Autodesk Inventor part; units mm, degrees
ref_plane "YZ Plane" through (0, 0, 0) normal (1, 0, 0) x (0, 1, 0)
ref_plane "XZ Plane" through (0, 0, 0) normal (0, 1, 0) x (-1, 0, 0)
ref_plane "XY Plane" through (0, 0, 0) normal (0, 0, 1) x (1, 0, 0)
sketch "Boceto1" plane through (0, 0, 0) normal (0, 1, 0) x (-1, 0, 0)
  line L0 (0, 0) -> (88.9, 0)
  line L1 (88.9, 0) -> (88.9, -139.7)
  line L2 (88.9, -139.7) -> (0, -139.7)
  line L3 (0, -139.7) -> (0, 0)
  circle A0 centre (60.325, -25.4) radius 3.9688
  circle A1 centre (60.325, -114.3) radius 3.9688
  circle A2 centre (28.575, -25.4) radius 3.9687
  circle A3 centre (28.575, -114.3) radius 3.9687
  line L4 (88.9, 0) -> (94.4562, 0)
  line L5 (94.4562, 0) -> (94.4562, -12.7)
  line L6 (94.4562, -12.7) -> (88.9, -12.7)
  line L7 (88.9, -12.7) -> (88.9, 0)
  line L8 (88.9, -139.7) -> (94.4563, -139.7)
  line L9 (94.4563, -139.7) -> (94.4563, -127)
  line L10 (94.4563, -127) -> (88.9, -127)
  line L11 (88.9, -127) -> (88.9, -139.7)
  line L12 (0, 0) -> (-5.5563, 0)
  line L13 (-5.5563, 0) -> (-5.5563, -12.7)
  line L14 (-5.5563, -12.7) -> (0, -12.7)
  line L15 (0, -12.7) -> (0, 0)
  line L16 (0, -139.7) -> (-5.5562, -139.7)
  line L17 (-5.5562, -139.7) -> (-5.5562, -127)
  line L18 (-5.5562, -127) -> (0, -127)
  line L19 (0, -127) -> (0, -139.7)
  line L20 (88.9, -63.5) -> (94.4562, -63.5)
  line L21 (94.4562, -63.5) -> (94.4562, -76.2)
  line L22 (94.4562, -76.2) -> (88.9, -76.2)
  line L23 (88.9, -76.2) -> (88.9, -63.5)
  line L24 (0, -63.5) -> (-5.5563, -63.5)
  line L25 (-5.5563, -63.5) -> (-5.5563, -76.2)
  line L26 (-5.5563, -76.2) -> (0, -76.2)
  line L27 (0, -76.2) -> (0, -63.5)
  dimension "d0" = 88.9
  dimension "d1" = 139.7
  dimension "d2" = 7.9375
  dimension "d3" = 7.9375
  dimension "d4" = 7.9375
  dimension "d5" = 7.9375
  dimension "d6" = 88.9
  dimension "d7" = 28.575
  dimension "d8" = 28.575
  dimension "d9" = 28.575
  dimension "d10" = 28.575
  dimension "d11" = 25.4
  dimension "d12" = 25.4
  dimension "d13" = 88.9
  dimension "d17" = 5.5563
  dimension "d18" = 12.7
  dimension "d19" = 5.5563
  dimension "d20" = 12.7
  dimension "d21" = 5.5563
  dimension "d22" = 12.7
  dimension "d23" = 5.5563
  dimension "d24" = 12.7
  dimension "d25" = 5.5563
  dimension "d26" = 12.7
  dimension "d27" = 5.5563
  dimension "d28" = 12.7
  dimension "d29" = 63.5
  dimension "d30" = 63.5
extrude "Extrusión1" add sketch "Boceto1" along normal blind 5
properties part number "CAR BOTTOM PLATE"
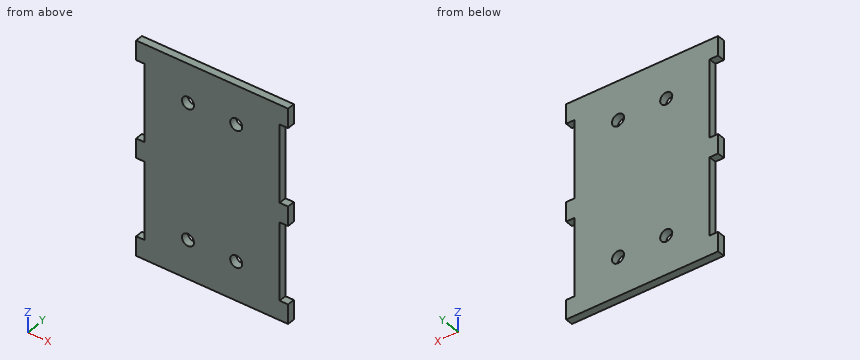
Model file for the job. Use its own axes, mm. Round coordinates to 2 decimals unless told otherwise and drop trailing zeros. Write each loop counter-clockwise with the first axis right and the second up, starting at its lowest first coordinate (ties: lowest second). Pieces come first, ordered by that corner, then holes. Notation, with made-up numbers: M -6.75,-37.5 L 48.25,-37.5 A12 cw 48.25,-28.5 Z; hole C 71.5,-36.75 d3. An arc over 180 degrees is marked long. Put each result on its own line as item: value.
Item 1: Flat gauge pins, fed straight in: P1, Ø2, axis at x = -21, y = 2, coming from the +Z side; P2, Ø1, axis at y = 3, z = -82, coming from the +X side; P3, Ø1, axis at y = 2, z = -52, coming from the -X side; P4, Ø6.5, axis at x = -28.575, z = -114.3, coming from the +Y side. Where does each tip first touch, or does it go through?
Responses:
P1: z = 0
P2: x = 0
P3: x = -88.9
P4: through
Item 2: Cut at A-A (z = -114.3). List the corners of the cut face in (x, y).
Responses:
outline: M -88.9,0 L -64.29,0 L -64.29,5 L -88.9,5 Z; M -56.36,0 L -32.54,0 L -32.54,5 L -56.36,5 Z; M -24.61,0 L 0,0 L 0,5 L -24.61,5 Z
Item 3: Probe L1, parallel to X at y = 0.3, z = -94.5; L2, parallel to Z at x = -57.5, y = 3.6. List the from-to ranges inside material, lowest first. Write a range as from..to.
Responses:
L1: -88.9..0
L2: -139.7..-117.09, -111.51..-28.19, -22.61..0
Item 4: Cut at B-B (z = -41.5). List the corners of the cut face in (x, y).
Responses:
outline: M -88.9,0 L 0,0 L 0,5 L -88.9,5 Z
